from build123d import *

# Parameters (mm, degrees)
BODY_DEPTH                      = 3.1
CHANNEL_W                       = 7.3
CHANNEL_H                       = 72
PIGIONCHANNEL_DEPTH             = 4.4
SKIZZE2_R                       = 1.75
SCREWS_DEPTH                    = 49.828144706
VERRUNDUNG1_R                   = 3
VERRUNDUNG2_R                   = 1
VERRUNDUNG3_R                   = 3
SKIZZE6_W                       = 19.5
SKIZZE6_H                       = 10
HANDLE_DEPTH                    = 10
SKIZZE7_R                       = 1.75
SCHNITT_LINEAR_AUSTRAGEN3_DEPTH = 52.800082742
SKIZZE8_W                       = 10
SKIZZE8_H                       = 8.274086909
SCHNITT_LINEAR_AUSTRAGEN4_DEPTH = 3.5
VERRUNDUNG7_R                   = 3
VERRUNDUNG8_R                   = 3
VERRUNDUNG12_R                  = 3
VERRUNDUNG13_R                  = 3
VERRUNDUNG14_R                  = 3
VERRUNDUNG16_R                  = 2
SKIZZE9_R                       = 9.5
GEAR_CAGE_DEPTH                 = 4.4
SCHNITT_LINEAR_AUSTRAGEN6_DEPTH = 4.4
VERRUNDUNG17_R                  = 2
SKIZZE11_W                      = 3
SKIZZE11_H                      = 54.597729832
SCHNITT_LINEAR_AUSTRAGEN7_DEPTH = 4.4
VERRUNDUNG18_R                  = 3
VERRUNDUNG19_R                  = 0.5
VERRUNDUNG20_START              = -4
VERRUNDUNG20_DEPTH              = 10.628110602
VERRUNDUNG22_START              = -3.1
VERRUNDUNG22_DEPTH              = 6.2


with BuildPart() as part:
    # body_sketch → body (new, symmetric)
    with BuildSketch(Plane.XY):
        Polygon((0, -35.644151565), (0, 36.355848435), (32, 36.355848435), (32, -13.644151565), (17, -13.644151565), (17, -35.644151565), align=None)
    extrude(amount=BODY_DEPTH, both=True)

    # channel → pigionchannel (cut)
    with BuildSketch(Plane.XY.offset(3.1)):
        with Locations((10.9, 0.355848435)):
            Rectangle(CHANNEL_W, CHANNEL_H)
    extrude(amount=-PIGIONCHANNEL_DEPTH, mode=Mode.SUBTRACT)

    # Skizze2 → screws (cut, through all)
    with BuildSketch(Plane.XY.offset(3.1)):
        with Locations((3.5, 32.855848435)):
            Circle(SKIZZE2_R)
        with Locations((28.5, 32.855848435)):
            Circle(SKIZZE2_R)
        with Locations((28.5, -10.144151565)):
            Circle(SKIZZE2_R)
        with Locations((2.8, -32.844151565)):
            Circle(SKIZZE2_R)
    extrude(amount=-SCREWS_DEPTH, mode=Mode.SUBTRACT)

    # Verrundung1
    verrundung1_edges = [part.edges().sort_by_distance(p)[0] for p in [
        (0, 36.355848435, 0),
        (32, 36.355848435, 0),
    ]]
    fillet(verrundung1_edges, radius=VERRUNDUNG1_R)

    # Verrundung2
    verrundung2_edges = [part.edges().sort_by_distance(p)[0] for p in [
        (14.55, 36.355848435, 0.9),
        (10.9, 36.355848435, -1.3),
        (7.25, 36.355848435, 0.9),
    ]]
    fillet(verrundung2_edges, radius=VERRUNDUNG2_R)

    # Verrundung3
    verrundung3_edges = [part.edges().sort_by_distance(p)[0] for p in [
        (32, -13.644151565, 0),
    ]]
    fillet(verrundung3_edges, radius=VERRUNDUNG3_R)

    # Skizze6 → handle (add)
    with BuildSketch(Plane.XZ.offset(35.644151565)):
        with Locations((13.75, 1.9)):
            Rectangle(SKIZZE6_W, SKIZZE6_H)
    extrude(amount=HANDLE_DEPTH)

    # Skizze7 → Schnitt-Linear austragen3 (cut, through all)
    with BuildSketch(Plane(origin=(23.5, 0, 0), x_dir=(0, 0, -1), z_dir=(1, 0, 0))):
        with Locations((-2.9, -41.644151565)):
            Circle(SKIZZE7_R)
    extrude(amount=-SCHNITT_LINEAR_AUSTRAGEN3_DEPTH, mode=Mode.SUBTRACT)

    # Skizze8 → Schnitt-Linear austragen4 (cut)
    with BuildSketch(Plane.ZY.offset(-4)):
        with Locations((1.9, -41.50710811)):
            Rectangle(SKIZZE8_W, SKIZZE8_H)
    extrude(amount=-SCHNITT_LINEAR_AUSTRAGEN4_DEPTH, mode=Mode.SUBTRACT)

    # Verrundung7
    verrundung7_edges = [part.edges().sort_by_distance(p)[0] for p in [
        (15.5, -45.644151565, 6.9),
    ]]
    fillet(verrundung7_edges, radius=VERRUNDUNG7_R)

    # Verrundung8
    verrundung8_edges = [part.edges().sort_by_distance(p)[0] for p in [
        (15.5, -45.644151565, -3.1),
    ]]
    fillet(verrundung8_edges, radius=VERRUNDUNG8_R)

    # Verrundung12
    verrundung12_edges = [part.edges().sort_by_distance(p)[0] for p in [
        (17, -13.644151565, 0),
    ]]
    fillet(verrundung12_edges, radius=VERRUNDUNG12_R)

    # Verrundung13
    verrundung13_edges = [part.edges().sort_by_distance(p)[0] for p in [
        (17, -35.644151565, 0),
    ]]
    fillet(verrundung13_edges, radius=VERRUNDUNG13_R)

    # Verrundung14
    verrundung14_edges = [part.edges().sort_by_distance(p)[0] for p in [
        (0, -35.644151565, 0),
    ]]
    fillet(verrundung14_edges, radius=VERRUNDUNG14_R)

    # Verrundung16
    verrundung16_edges = [part.edges().sort_by_distance(p)[0] for p in [
        (14.55, -35.644151565, 0.9),
        (7.25, -35.644151565, 0.9),
    ]]
    fillet(verrundung16_edges, radius=VERRUNDUNG16_R)

    # Skizze9 → gear cage (cut)
    with BuildSketch(Plane.XY.offset(3.1)):
        with Locations((20.75, 23.105848435)):
            Circle(SKIZZE9_R)
    extrude(amount=-GEAR_CAGE_DEPTH, mode=Mode.SUBTRACT)

    # Skizze10 → Schnitt-Linear austragen6 (cut)
    with BuildSketch(Plane.XY.offset(3.1)):
        Polygon((16.55, 11.83128846), (30, 11.83128846), (30, -6.16871154), (25.418135465, -6.16871154), (25.418135465, -11.465988975), (16.55, -11.465988975), align=None)
    extrude(amount=-SCHNITT_LINEAR_AUSTRAGEN6_DEPTH, mode=Mode.SUBTRACT)

    # Verrundung17
    verrundung17_edges = [part.edges().sort_by_distance(p)[0] for p in [
        (25.418135465, -6.16871154, 0.9),
    ]]
    fillet(verrundung17_edges, radius=VERRUNDUNG17_R)

    # Skizze11 → Schnitt-Linear austragen7 (cut)
    with BuildSketch(Plane.XY.offset(3.1)):
        with Locations((3.5, 1.149247054)):
            Rectangle(SKIZZE11_W, SKIZZE11_H)
    extrude(amount=-SCHNITT_LINEAR_AUSTRAGEN7_DEPTH, mode=Mode.SUBTRACT)

    # Verrundung18
    verrundung18_edges = [part.edges().sort_by_distance(p)[0] for p in [
        (13.75, -35.644151565, 6.9),
        (23.5, -35.644151565, 1.9),
    ]]
    fillet(verrundung18_edges, radius=VERRUNDUNG18_R)

    # Verrundung19
    verrundung19_edges = [part.edges().sort_by_distance(p)[0] for p in [
        (7.5, -37.370064656, 1.758004285),
    ]]
    fillet(verrundung19_edges, radius=VERRUNDUNG19_R)

    # Verrundung20: read off the stored shape, not the designer's step
    # Verrundung20 outline → Verrundung20 (cut)
    with BuildSketch(Plane.XY.offset(VERRUNDUNG20_START)):
        with BuildLine():
            ThreePointArc((7, -37.370064656), (7.080813571, -37.376638707), (7.159502052, -37.396187989))
            ThreePointArc((7.159502052, -37.396187989), (5.499970333, -36.664033092), (3.999994229, -35.644146822))
            Line((3.999994229, -35.644146822), (4, -37.370064656))
            Line((4, -37.370064656), (7, -37.370064656))
        make_face()
    extrude(amount=VERRUNDUNG20_DEPTH, mode=Mode.SUBTRACT)

    # Verrundung22: read off the stored shape, not the designer's step
    # Verrundung22 outline → Verrundung22 (add)
    with BuildSketch(Plane.XY.offset(VERRUNDUNG22_START)):
        with BuildLine():
            ThreePointArc((2.557893696, -35.611396418), (4.007665984, -35.968268897), (5.36587668, -36.588318377))
            ThreePointArc((5.36587668, -36.588318377), (4.663304696, -36.144631367), (3.999994229, -35.644146822))
            Line((3.999994229, -35.644146822), (3, -35.644151565))
            ThreePointArc((3, -35.644151565), (2.778340981, -35.635951572), (2.557893696, -35.611396418))
        make_face()
    extrude(amount=VERRUNDUNG22_DEPTH)


solid = part.part
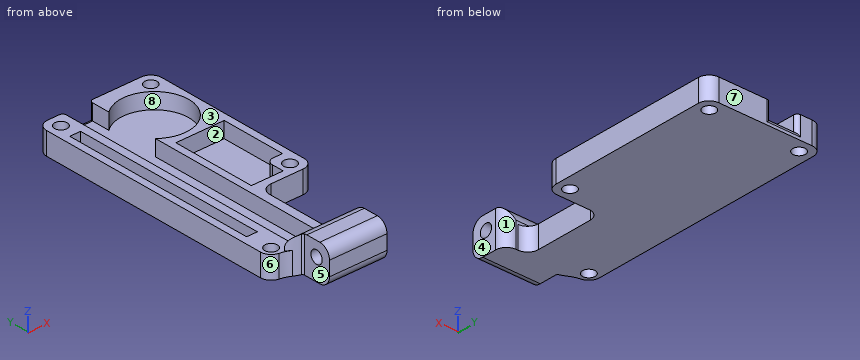
Can you work these out from the model? Positions are in its coordinate system, mm. Face numbers are marked on the shaded views. A direction names the side the tool comes from. Coordinates: 2 decimals unless noted, no trailing zeros. Write each loop counter-clockwise with the first axis right and the second up, starting at its lowest first coordinate (ties: lowest second). Pieces come first, ordered by that corner, then holes. Notation, with made-up numbers: (-16.5, 26) - (16.5, 26) arc R6 ccw to (16.5, 37) - close; hole circle Ø10 at (77, 21.5). An arc over 180 degrees is marked (long way). Return JSON: item names as keys, results as strings. Group by question number.
Item 1: If we section it at D-D (y = 27.5): Write out the boundary of the cut face in (x, z), then the cut area to 3 significant figures.
Item 2: Which directions (+Z, -Z, +X, -X, +Y, -Y) give clear straight access to the entire face, cutting with the end or side of a thin tool? Please do the marked faces 1, 2, 3, 4 and 5.
Item 3: Please list where these lines run through material, in increasing order: probe 1 along X at (y, z) = (-23, 1); probe 2 along X at (y, z) = (1.5, 0); probe 3 along Y at (x, z) = (20.75, 1).
Item 4: If we section it at A-A (y = -27): Write out the boundary of the cut face in (x, z).
Item 5: We'd pull the mould along X, two halves only. Please class the marked faces 6, 7 and 8: pulls with the +X half, pulls with the -X half, needs draft (parallel to the pull), parting line crosses it, or undercut.
Item 6: If we section it at C-C (y = 8): Write out the boundary of the cut face in (x, z), then the cut area to 3 significant figures.
Item 7: I'm going to push flat-ended pins straight in: pin 1 Ø2 at (x, z) = (21.5, 6) entering from +Y; pin 2 Ø2.5 at (x, z) = (3.5, 0) entering from -Y; pin 3 Ø2 at (y, z) = (-16, 0) entering from +X. Where does each tip first touch, or does it pass through?
Item 8: If we section it at B-B (z = 2): Count the separate pieces of the cut face and the enclosed holes in it, then the cut area to 3 significant figures.
Return value:
{
 "1": {"outline": "(0, -3.1) - (32, -3.1) - (32, 3.1) - (29.17, 3.1) - (29.17, -1.3) - (7.25, -1.3) - (7.25, 3.1) - (5, 3.1) - (5, -1.3) - (2, -1.3) - (2, 3.1) - (0, 3.1) - close", "area": "88.7 mm^2"},
 "2": {"face 1": "+Z, -Z, +X", "face 2": "+Z", "face 3": "+Z, +X, -X, +Y", "face 4": "+Z, -Z, +X, -Y", "face 5": "+Z, -Z, -X, -Y"},
 "3": {"probe 1": "x = 0 to 2, 5 to 7.25, 14.55 to 17", "probe 2": "x = 0 to 2, 5 to 7.25, 14.55 to 16.55, 30 to 32", "probe 3": "y = -45.64 to -35.65, -13.64 to -11.47, 11.83 to 13.61, 32.61 to 36.36"},
 "4": {"outline": "(0, -3.1) - (17, -3.1) - (17, 3.1) - (14.55, 3.1) - (14.55, -1.3) - (7.25, -1.3) - (7.25, 3.1) - (0, 3.1) - close"},
 "5": {"face 6": "pulls with the -X half", "face 7": "needs draft", "face 8": "undercut"},
 "6": {"outline": "(0, -3.1) - (32, -3.1) - (32, 3.1) - (30, 3.1) - (30, -1.3) - (16.55, -1.3) - (16.55, 3.1) - (14.55, 3.1) - (14.55, -1.3) - (7.25, -1.3) - (7.25, 3.1) - (5, 3.1) - (5, -1.3) - (2, -1.3) - (2, 3.1) - (0, 3.1) - close", "area": "93.9 mm^2"},
 "7": {"pin 1": "stops at y = -35.85", "pin 2": "stops at y = -36.27", "pin 3": "stops at x = 17.49"},
 "8": {"separate pieces": "2", "enclosed holes": "6", "area": "817 mm^2"}
}
